The model under review builds one solid part; all positions refer to its coordinate system, in mm. Face numbers are marked on the shaded views. A direction names the side the tool comes from. Round coordinates to 2 decimals unless told otherwise and drop trailing zeros. Write each loop counter-clockwise with the first axis right and the second up, starting at its lowest first coordinate (ties: lowest second). Pieces come first, ordered by that corner, then holes.
Item 1: Add section C-C (z = 7). Give the boundary of the cut face in (x, y).
Item 2: Add section B-B (y = 5). Give the boundary of the cut face in (x, z), plus the area to 3 significant figures.
Item 3: Add section D-D (y = -14.5). Give the boundary of the cut face in (x, z).
Item 4: Clearance check with flat-ended pins moving along their axes: pin 1 Ø18 at (x, y) = (0, 0) entering from -Z; pin 2 Ø2 at (x, z) = (21.5, 2) entering from -Y; pin 3 Ø4.5 at (x, z) = (-22, 2.5) entering from +Y; pin 4 Ø8 at (x, y) = (-26.5, 0.5) entering from +Z. State where each tip first meets the part, or that it passes through.
Item 5: Machinability: for the marked faces 5, 6 and 7, which of the approach directions +Z, -Z, +X, -X, +Y, -Y give a long, thin tool a straight path to every point of the face, cutting with its end or side? Answer none if there is none.
Item 6: To check wall thickness, follow L1, parallel to X at y = 0, z = 3.25; L2, parallel to Y at x = 0, z = 7.5; L3, parallel to Y at x = -27.5, z = 0.4. State the ranges of each line that lie inside material, in increasing order.
Item 7: Add section A-A (x = -6). Give the boundary of the cut face in (y, z), plus the area to 3 significant figures.
Item 8: Draft analysis for pull direction X (two halves, no side actions). For the marked faces 1, 2, 3 and 4, state which applies: +X half, -X half, draft (parallel to the pull), parting line (faces both ways), or undercut.
```python
from build123d import *

# Parameters (mm, degrees)
PAD_DEPTH       = 4
SKETCH001_R     = 2.25
HOLE_DEPTH      = 4.001
POCKET001_DEPTH = 3
SKETCH002_R     = 10
POCKET_DEPTH    = 11.501


with BuildPart() as part:
    # Sketch → Pad (new body)
    with BuildSketch(Plane.XY):
        with BuildLine():
            ThreePointArc((-27.5, 7.5), (-35, 0), (-27.5, -7.5))
            Line((-16.911535, -7.5), (-27.5, -7.5))
            ThreePointArc((-16.911535, -7.5), (0, -18.5), (16.911535, -7.5))
            Line((27.5, -7.5), (16.911535, -7.5))
            ThreePointArc((27.5, -7.5), (35, 0), (27.5, 7.5))
            Line((27.5, 7.5), (16.911535, 7.5))
            ThreePointArc((16.911535, 7.5), (0, 18.5), (-16.911535, 7.5))
            Line((-27.5, 7.5), (-16.911535, 7.5))
        make_face()
    extrude(amount=PAD_DEPTH)

    # Sketch001 (on DatumPlane) → Hole (cut, through all)
    with BuildSketch(Plane.XY.offset(4)):
        with Locations((-27.5, 0)):
            Circle(SKETCH001_R)
        with Locations((27.5, 0)):
            Circle(SKETCH001_R)
    extrude(amount=-HOLE_DEPTH, mode=Mode.SUBTRACT)

    # Sketch003 → Revolution (revolve)
    with BuildSketch(Plane.XZ):
        Polygon((0, 4), (-13.55, 4), (-13.55, 5.5), (-12.55, 5.5), (-12.55, 11.5), (0, 11.5), align=None)
    revolve(axis=Axis((0, 0, 0), (0, 0, 1)))

    # Sketch004 (on DatumPlane) → Pocket001 (cut)
    with BuildSketch(Plane.XY.offset(4)):
        Polygon((-23.169873, 0), (-25.334936, 3.75), (-29.665064, 3.75), (-31.830127, 0), (-29.665064, -3.75), (-25.334936, -3.75), align=None)
        Polygon((31.830127, 0), (29.665064, 3.75), (25.334936, 3.75), (23.169873, 0), (25.334936, -3.75), (29.665064, -3.75), align=None)
    extrude(amount=-POCKET001_DEPTH, mode=Mode.SUBTRACT)

    # Sketch002 → Pocket (cut, through all)
    with BuildSketch(Plane.XY):
        Circle(SKETCH002_R)
    extrude(amount=POCKET_DEPTH, mode=Mode.SUBTRACT)


solid = part.part
```
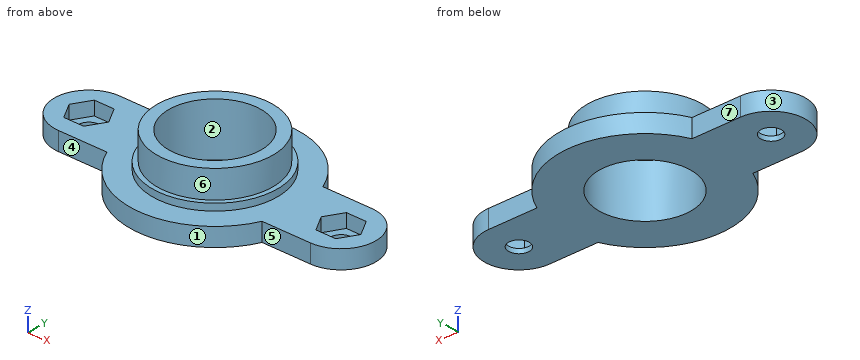
Numbers:
1. outline: circle Ø25.1 at (0, 0); hole circle Ø20 at (0, 0)
2. outline: (-33.09, 0) - (-8.66, 0) - (-8.66, 11.5) - (-11.51, 11.5) - (-11.51, 5.5) - (-12.59, 5.5) - (-12.59, 4) - (-33.09, 4) - close; (8.66, 0) - (33.09, 0) - (33.09, 4) - (12.59, 4) - (12.59, 5.5) - (11.51, 5.5) - (11.51, 11.5) - (8.66, 11.5) - close
2. area: 241 mm2
3. outline: (-11.49, 0) - (11.49, 0) - (11.49, 4) - (-11.49, 4) - close
4. pin 1: passes through
4. pin 2: stops at y = -7.5
4. pin 3: stops at y = 7.5
4. pin 4: stops at z = 4
5. face 5: +Z, -Z, +X, -Y
5. face 6: +Z
5. face 7: +Z, -Z, -X, +Y
6. L1: x = -35 to -31.83, -23.17 to -10, 10 to 23.17, 31.83 to 35
6. L2: y = -12.55 to -10, 10 to 12.55
6. L3: y = -7.5 to -2.25, 2.25 to 7.5
7. outline: (-17.5, 0) - (-8, 0) - (-8, 11.5) - (-11.02, 11.5) - (-11.02, 5.5) - (-12.15, 5.5) - (-12.15, 4) - (-17.5, 4) - close; (8, 0) - (17.5, 0) - (17.5, 4) - (12.15, 4) - (12.15, 5.5) - (11.02, 5.5) - (11.02, 11.5) - (8, 11.5) - close
7. area: 125 mm2
8. face 1: parting line
8. face 2: undercut
8. face 3: -X half
8. face 4: draft
